from build123d import *

# Parameters (mm, degrees)
F0_W      = 52.4510033429
F0_H      = 54.2289987206
F2_DEPTH  = 25.4
F3_W      = 52.4510033429
F3_H      = 9.7890347242
F4_DEPTH  = 65.024
F5_W      = 12.0777860284
F5_H      = 18.1565545499
F6_DEPTH  = 50.8
F7_DEPTH  = 12.7
F8_DEPTH  = 12.446
F9_DEPTH  = 27.686
F10_W     = 11.244142428
F10_H     = 31.9378077536
F10_H_2   = 5.1374584885
F11_DEPTH = 65.278


with BuildPart() as f2:
    # F0 (on Top) → F2 (new body)
    with BuildSketch(Plane.XY):
        with BuildLine():
            ThreePointArc((-26.2255016714, -27.1144993603), (0, -53.3400010318), (26.2255016714, -27.1144993603))
            Line((26.2255016714, -27.1144993603), (-26.2255016714, -27.1144993603))
        make_face()
        Rectangle(F0_W, F0_H)
    extrude(amount=F2_DEPTH)

    # F3 (on face) → F4 (join)
    with BuildSketch(Plane.XY.offset(25.4)):
        with Locations((0, 22.2199819982)):
            Rectangle(F3_W, F3_H)
    extrude(amount=F4_DEPTH)

    # F5 (on face) → F6 (cut)
    with BuildSketch(Plane.XY):
        with Locations((20.1866086572, 18.0362220854)):
            Rectangle(F5_W, F5_H)
    extrude(amount=F6_DEPTH, mode=Mode.SUBTRACT)

    # F7 (cut): a face of the model
    f7_faces = [f2.faces().sort_by_distance(p)[0] for p in [
        (-0.6162983013, -16.3297638345, 25.4),
    ]]
    extrude(f7_faces, amount=-F7_DEPTH, mode=Mode.SUBTRACT)

    # F8 (cut): a face of the model
    f8_faces = [f2.faces().sort_by_distance(p)[0] for p in [
        (0, 22.2199819982, 90.424),
    ]]
    extrude(f8_faces, amount=-F8_DEPTH, mode=Mode.SUBTRACT)

    # F9 (add): a face of the model
    f9_faces = [f2.faces().sort_by_distance(p)[0] for p in [
        (20.1866086572, 22.2199819982, 50.8),
    ]]
    extrude(f9_faces, amount=F9_DEPTH)

    # F10 (on face) → F11 (cut)
    with BuildSketch(Plane.XZ.offset(-17.3254646361)):
        with Locations((0, 62.0090961232)):
            Rectangle(F10_W, F10_H)
        with BuildLine():
            ThreePointArc((-5.622071214, 46.0401922464), (0, 40.4181210324), (5.622071214, 46.0401922464))
            Line((5.622071214, 46.0401922464), (-5.622071214, 46.0401922464))
        make_face()
        with Locations((0, 80.5467292442)):
            Rectangle(F10_W, F10_H_2)
    extrude(amount=-F11_DEPTH, mode=Mode.SUBTRACT)


solid = f2.part
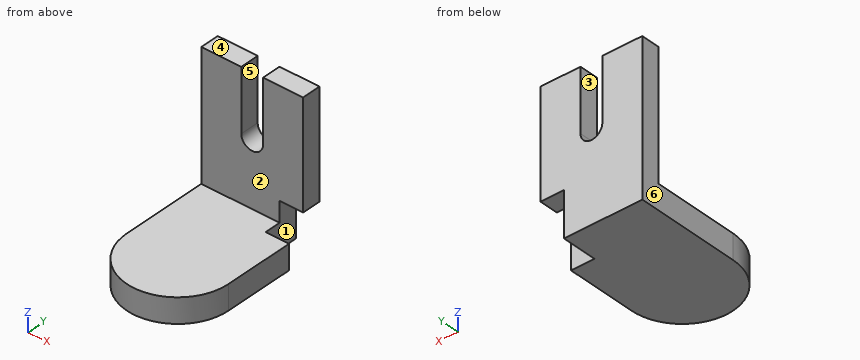
Work out the finished part from the listing and answer in its coordinate system (mm). Face numbers are marked on the shaded views. A direction names the side the tool comes from. Round coordinates to 2 decimals unless told otherwise and drop trailing zeros. Write each loop counter-clockwise with the first axis right and the second up, starting at its lowest first coordinate (ties: lowest second). Pieces come first, ordered by that corner, then holes. Notation, with made-up numbers: (8, 50.25) - (22, 50.25) arc R22 ccw to (22, 63.25) - close; hole circle Ø8 at (71, 40.25). An arc over 180 degrees is marked (long way). Answer in a Markdown table with one row per item. Add a question column.
1. A cutting plane is placed at D-D, the plane x = 0. Determine the outline of the cut face in (y, z), and give its area (3 significant figures).
2. A cutting plane is placed at C-C, the plane y = 21. Determine the outline of the cut face in (x, z), and give its area (3 significant figures).
3. For the marked faces 1, 2 and 3, determine the directions among +Z, -Z, +X, -X, +Y, -Y from which every point of the face is accessible in a straight line to the end or side of a thin tool.
4. Find the intervals of material crossed by line 1 along Y through (x, z) = (-9.5, 32.5); line 2 along Z through (x, y) = (3.5, -23.5); line 3 along Y through (x, z) = (-23.5, 7), in increasing order. Write a range as from..to.
5. The mould has two halves that part along X. Classify the marked faces 4, 5 and 6: +X half, -X half, draft (parallel to the pull), parting line (faces both ways), or undercut.
6. Given pin 1 (6 mm diameter, centred on x = 21, y = -3.5, fed in from +Z); pin 2 (5.5 mm diameter, centred on y = 21.5, z = 7, fed in from +X); pin 3 (9.5 mm diameter, centred on x = 22, z = 9, fed in from +Y), each flat-ended and moving along its own axis, determine where each tip first touches the part or whether it passes through.
7. A cutting plane is placed at A-A, the plane z = 69.5. Determine the outline of the cut face in (x, y), and give its area (3 significant figures).
8. A cutting plane is placed at B-B, the plane x = 16. Determine the outline of the cut face in (y, z).
Worked out:
| question | item | result |
|---|---|---|
| 1 | outline | (-53.34, 0) - (27.11, 0) - (27.11, 40.42) - (17.33, 40.42) - (17.33, 12.7) - (-53.34, 12.7) - close |
| 1 | area | 1,290 mm^2 |
| 2 | outline | (-26.23, 0) - (14.15, 0) - (14.15, 23.11) - (26.23, 23.11) - (26.23, 77.98) - (5.62, 77.98) - (5.62, 46.04) arc R5.62 cw to (-5.62, 46.04) - (-5.62, 77.98) - (-26.23, 77.98) - close |
| 2 | area | 3,400 mm^2 |
| 3 | face 1 | -Z, +X, +Y |
| 3 | face 2 | +Z, +X, -X, -Y |
| 3 | face 3 | +Z, +Y, -Y |
| 4 | line 1 | 17.33..27.11 |
| 4 | line 2 | 0..12.7 |
| 4 | line 3 | -38.76..27.11 |
| 5 | face 4 | draft |
| 5 | face 5 | undercut |
| 5 | face 6 | -X half |
| 6 | pin 1 | z = 12.7 |
| 6 | pin 2 | x = 14.15 |
| 6 | pin 3 | y = 8.96 |
| 7 | outline | (-26.23, 17.33) - (-5.62, 17.33) - (-5.62, 27.11) - (-26.23, 27.11) - close; (5.62, 17.33) - (26.23, 17.33) - (26.23, 27.11) - (5.62, 27.11) - close |
| 7 | area | 403 mm^2 |
| 8 | outline | (-47.89, 0) - (8.96, 0) - (8.96, 12.7) - (-47.89, 12.7) - close; (17.33, 23.11) - (27.11, 23.11) - (27.11, 77.98) - (17.33, 77.98) - close |
